Input: part model. Units: mm. Frame: model coordinates. Face numbers are marked on the shaded views. Give positions to 0.01 mm unless a question says otherwise; leave off trailing zeros. Answer in a Markdown table with one row per item. Add a question column.
```python
from build123d import *

# Parameters (mm, degrees)
FILLET1_R       = 1.3
RECPAT_COUNT    = 2
RECPAT_ANGLE    = 90
THDSCHPAT_COUNT = 22
THDSCHPAT_PITCH = 0.785714286


with BuildPart() as part:
    # BodySke → Base-Revolve (revolve)
    with BuildSketch(Plane.XY, mode=Mode.PRIVATE) as base_revolve_sk:
        Polygon((0, 0), (0, 4.65), (0.55, 4.65), (2.7, 2.5), (20, 2.5), (20, 0), align=None)
    revolve(base_revolve_sk.sketch.rotate(Axis((-6.35, 0, 0), (1, 0, 0)), 90), axis=Axis((-6.35, 0, 0), (1, 0, 0)))

    # Fillet1
    fillet1_edges = [part.edges().sort_by_distance(p)[0] for p in [
        (2.7, 0, -2.5),
    ]]
    fillet(fillet1_edges, radius=FILLET1_R)

    # Sketch3 → Recess section 0
    with BuildSketch(Plane.ZY):
        with BuildLine():
            Line((-0.515, 2.45), (0.515, 2.45))
            Line((0.515, 2.45), (0.515, -2.45))
            Line((0.515, -2.45), (-0.515, -2.45))
            Line((-0.515, -2.45), (-0.515, 2.45))
        make_face()
    # Sketch4 → Recess section 1
    with BuildSketch(Plane.ZY.offset(-3.05)):
        with BuildLine():
            Line((-0.515, 0.92932635), (0.515, 0.92932635))
            Line((0.515, 0.92932635), (0.515, -0.92932635))
            Line((0.515, -0.92932635), (-0.515, -0.92932635))
            Line((-0.515, -0.92932635), (-0.515, 0.92932635))
        make_face()
    recess = loft(mode=Mode.SUBTRACT)

    # RecPat: Recess ×2 about axis
    recpat_axis = Axis((0, 0, 0), (1, 0, 0))
    for i in range(1, RECPAT_COUNT):
        add(recess.rotate(recpat_axis, i * RECPAT_ANGLE / (RECPAT_COUNT - 1)), mode=Mode.SUBTRACT)

    # RecCorSke → RecessCore (revolve, cut)
    with BuildSketch(Plane.XY, mode=Mode.PRIVATE) as recesscore_sk:
        Polygon((0, 0), (0, 1.064276776), (3.05, 0.851), (3.326506661, 0), align=None)
    revolve(recesscore_sk.sketch.rotate(Axis((-3.175, 0, 0), (1, 0, 0)), 90), axis=Axis((-3.175, 0, 0), (1, 0, 0)), mode=Mode.SUBTRACT)

    # ThdSchSke → ThreadSchematic (revolve, cut)
    with BuildSketch(Plane.XY):
        Polygon((3.500001, -2.055), (3.188408645, -2.5), (3.188408645, -3.125), (3.811593355, -3.125), (3.811593355, -2.5), align=None)
    threadschematic = revolve(axis=Axis((-3.175, 0, 0), (1, 0, 0)), mode=Mode.SUBTRACT)

    # ThdSchPat: ThreadSchematic ×22
    with Locations(*[(i * THDSCHPAT_PITCH, 0, 0) for i in range(1, THDSCHPAT_COUNT)]):
        add(threadschematic, mode=Mode.SUBTRACT)


solid = part.part
```
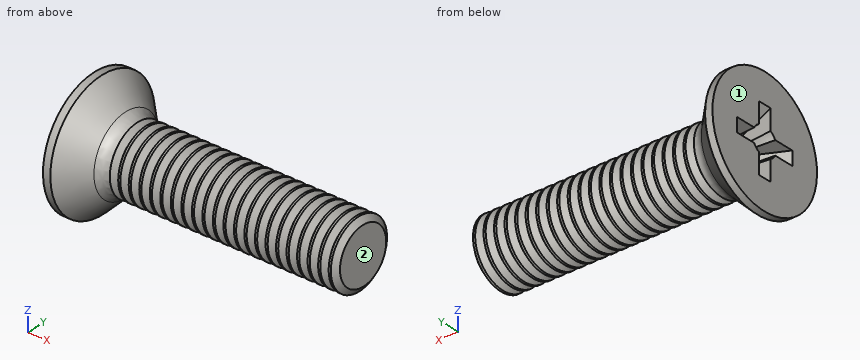
1) Material intervals for line 1 along Z through (x, y) = (3, 0.25); line 2 along Y through (x, z) = (1.5, 1.5) (3 decimals); line 3 along Z through (x, y) = (2.5, 0.25), sorted ascending.
2) Pull-direction query (X, two-part tool) for the marked faces 1 and 2; classes: +X half, -X half, draft (parallel to the pull), parting line (faces both ways), or undercut.
3) Pin query (flat end, axial travel): pin 1 (1.5 mm diameter, centred on x = 9.5, z = 1, fed in from -Y); pin 2 (1 mm diameter, centred on y = 2, z = 3, fed in from +X); pin 3 (2 mm diameter, centred on x = 10.5, y = -1, fed in from -Z); pin 4 (4 mm diameter, centred on y = 3.5, z = -0.5, fed in from -X). Return the tip coordinate at first contact, or that it passes through.
Working result:
| question | item | result |
|---|---|---|
| 1 | line 1 | z = -2.51 to -0.95, 0.95 to 2.51 |
| 1 | line 2 | y = -3.382 to -0.515, 0.515 to 3.382 |
| 1 | line 3 | z = -2.72 to -1.2, 1.2 to 2.72 |
| 2 | face 1 | -X half |
| 2 | face 2 | +X half |
| 3 | pin 1 | stops at y = -2.49 |
| 3 | pin 2 | stops at x = 2.09 |
| 3 | pin 3 | stops at z = -2.5 |
| 3 | pin 4 | stops at x = 0 |
